Could you check a few things on this drawing? It's one solid part, dimensions in mm from its lowest x, y, z. A direction names the side the tool comes from. Give positions to 0.01 mm unless a question says otherwise; leave off trailing zeros. Order: outer loops, then holes, each group sorted by start corner. A loop starts at its lowest first (then second) coordinate and runs counter-clockwise, first axis right, second up. Notation, with made-up numbers: (-38, 13.5) -> (-16, 13.5) arc R34 ccw to (-16, 49.5) -> close; hole circle Ø8 at (6.5, -28.5). An arc over 180 degrees is marked (long way). Write each question's results on one line, items separated by ' | '. Start each with the question number.
Q1. Imagine slicing it at B-B, the plane x = 55. Please give me the cut outline in (y, z), then the cut area to 3 significant figures.
Q2. Imagine slicing it at D-D, the plane y = 28.5. Please give me the cut outline in (x, z), then the cut area to 3 significant figures.
Q3. I'm going to push flat-ended pins straight in: pin 1 (8 mm diameter, centred on y = 74.5, z = 32.5, fed in from +X); pin 2 (3 mm diameter, centred on y = 75.5, z = 21.5, fed in from -X); pin 3 (15 mm diameter, centred on x = 59.5, z = 18, fed in from -Y). Where does each tip first touch, or does it pass through?
Q4. For the marked faces 1, 2 and 3, which set-ups out of +Z, -Z, +X, -X, +Y, -Y let a thin tool reach every point of the face, with its end or its side?
Q5. Imagine slicing it at A-A, the plane z = 15.5. Please give me the cut outline in (x, y).
Q6. I need wall thicknesses on line 1 along X through (y, z) = (55.5, 24.5); line 2 along Z through (x, y) = (2.95, 45); line 3 along Z through (x, y) = (55, 74.25). Which ranges of each line are inside material? Lowest first, please. Write a range as [from, to].
Q7. Thinking about a two-plate mould opening in X: for the marked faces 4, 5 and 6, which applies, pulls with the +X half, pulls with the -X half, needs draft (parallel to the pull), parting line crosses it, or undercut?
Q8. Imagine slicing it at C-C, the plane y = 45. Please give me the cut outline in (x, z), then the cut area to 3 significant figures.
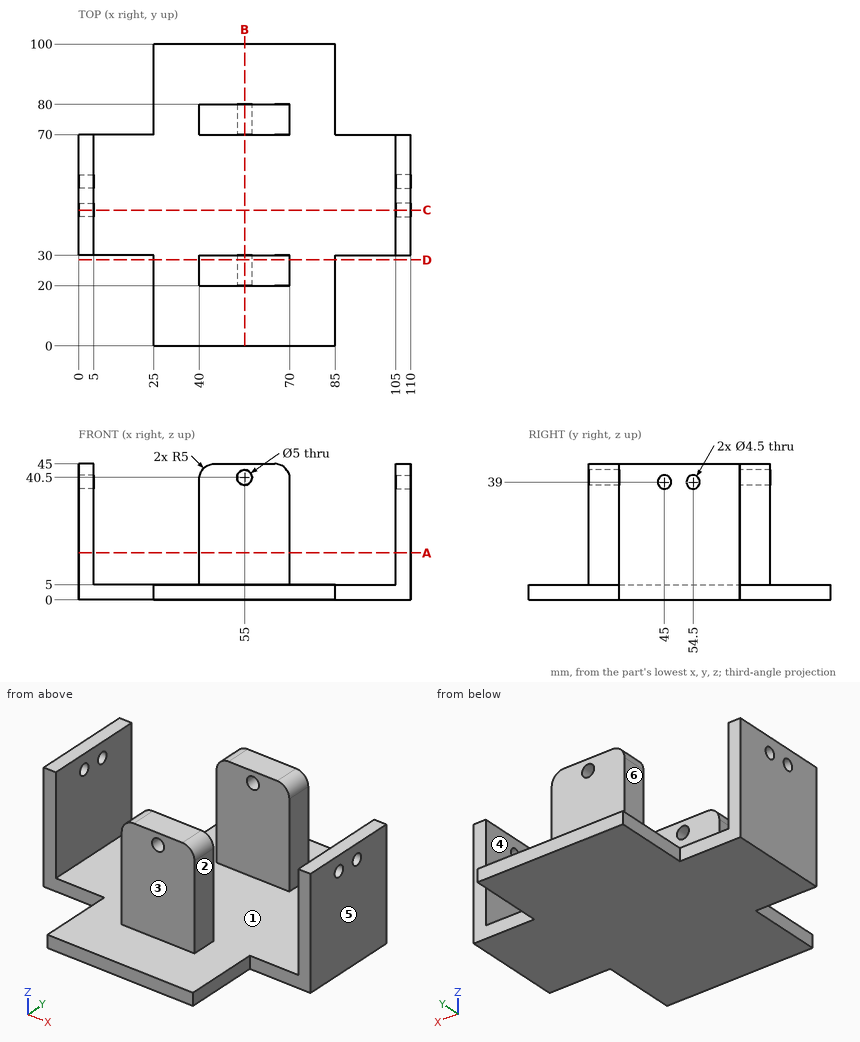
Geometry check:
1) outline: (0, 0) -> (100, 0) -> (100, 5) -> (80, 5) -> (80, 38) -> (70, 38) -> (70, 5) -> (30, 5) -> (30, 38) -> (20, 38) -> (20, 5) -> (0, 5) -> close; (20, 43) -> (30, 43) -> (30, 45) -> (20, 45) -> close; (70, 43) -> (80, 43) -> (80, 45) -> (70, 45) -> close | area: 1,200 mm²
2) outline: (25, 0) -> (85, 0) -> (85, 5) -> (70, 5) -> (70, 40) arc R5 ccw to (65, 45) -> (45, 45) arc R5 ccw to (40, 40) -> (40, 5) -> (25, 5) -> close; hole circle Ø5 at (55, 40.5) | area: 1,470 mm²
3) pin 1: x = 70 | pin 2: x = 40 | pin 3: y = 20
4) face 1: +Z | face 2: +Z, +X, +Y, -Y | face 3: +Z, +X, -X, -Y
5) outline: (0, 30) -> (5, 30) -> (5, 70) -> (0, 70) -> close; (40, 20) -> (70, 20) -> (70, 30) -> (40, 30) -> close; (40, 70) -> (70, 70) -> (70, 80) -> (40, 80) -> close; (105, 30) -> (110, 30) -> (110, 70) -> (105, 70) -> close
6) line 1: [0, 5], [105, 110] | line 2: [0, 36.75], [41.25, 45] | line 3: [0, 38], [43, 45]
7) face 4: undercut | face 5: pulls with the +X half | face 6: pulls with the -X half
8) outline: (0, 0) -> (110, 0) -> (110, 36.75) -> (105, 36.75) -> (105, 5) -> (5, 5) -> (5, 36.75) -> (0, 36.75) -> close; (0, 41.25) -> (5, 41.25) -> (5, 45) -> (0, 45) -> close; (105, 41.25) -> (110, 41.25) -> (110, 45) -> (105, 45) -> close | area: 905 mm²
